from build123d import *

# Parameters (mm, degrees)
ESQUISSE1_W             = 150
ESQUISSE1_H             = 150
BOSS_EXTRU_1_DEPTH      = 250
CONG_1_R                = 20
ESQUISSE2_W             = 60
ESQUISSE2_H             = 80
ENL_V_MAT_EXTRU_1_DEPTH = 40
ESQUISSE4_W             = 60
ESQUISSE4_H             = 60
ENL_V_MAT_EXTRU_2_DEPTH = 40


with BuildPart() as part:
    # Esquisse1 → Boss.-Extru.1 (new body)
    with BuildSketch(Plane.XY):
        with Locations((75, 75)):
            Rectangle(ESQUISSE1_W, ESQUISSE1_H)
    extrude(amount=BOSS_EXTRU_1_DEPTH)

    # Congé1
    cong_1_edges = [part.edges().sort_by_distance(p)[0] for p in [
        (150, 75, 250),
        (75, 150, 250),
        (0, 75, 250),
        (75, 150, 0),
        (150, 75, 0),
        (75, 0, 0),
        (0, 75, 0),
        (0, 150, 125),
        (150, 150, 125),
        (150, 0, 125),
        (0, 0, 125),
        (75, 0, 250),
    ]]
    fillet(cong_1_edges, radius=CONG_1_R)

    # Esquisse2 → Enlèv. mat.-Extru.1 (cut)
    with BuildSketch(Plane(origin=(150, 0, 0), x_dir=(0, 0, -1), z_dir=(1, 0, 0))):
        with Locations((-105.364762055, 20.069300744)):
            Rectangle(ESQUISSE2_W, ESQUISSE2_H)
    extrude(amount=-ENL_V_MAT_EXTRU_1_DEPTH, mode=Mode.SUBTRACT)

    # Esquisse4 → Enlèv. mat.-Extru.2 (cut)
    with BuildSketch(Plane.ZY):
        with Locations((105.517882432, 30)):
            Rectangle(ESQUISSE4_W, ESQUISSE4_H)
    extrude(amount=-ENL_V_MAT_EXTRU_2_DEPTH, mode=Mode.SUBTRACT)


solid = part.part
Geometry: final body of the model. Coordinates: model frame, mm. A direction names the side the tool comes from. Give positions to 0.01 mm unless a question says otherwise; leave off trailing zeros. Loops run counter-clockwise (first coordinate to the right, second up) from the corner with the lowest first, then second, coordinate; pieces in that order, holes last. Notation, with made-up numbers: (88.25, 86) - (117.25, 86) arc R34 ccw to (117.25, 122) - close; hole circle Ø6 at (50.5, 66). An arc over 180 degrees is marked (long way). One line per question, with ' | ' between items. Start each with the question number.
(1) Ray query, line 1 (Z direction, x = 38, y = 41); line 2 (X direction, y = 14, z = 77); line 3 (Z direction, x = 15, y = 16). Return the intervals inside material, ascending. Write a range as from..to.
(2) Pull-direction query (Z, two-part tool) for faces 3 (the flat face through (74, 0, 124)), 4 (the flat face through (130, 30, 75.365)), 5 (the cylindrical face through (75.77, 5.703, 6.014)); classes: released by +Z, released by -Z, zero draft, split by the parting line, or undercut.
(3) Contact query for flat-ended pins moving along their axis: pin 1 (12 mm diameter, centred on x = 16.5, z = 93, fed in from -Y); pin 2 (1 mm diameter, centred on x = 77.5, y = 18.5, fed in from -Z) (3 decimals). Output: stop coordinate, or through.
(4) Section query D-D on z = 169.5. Return loops of the section in (x, y).
(5) Reachability of faces 1 (the flat face through (110, 30, 106)), 2 (the cylindrical face through (143.986, 5.703, 183.345)) from +Z, -Z, +X, -X, +Y, -Y: full face, straight path, thin tool, end or side. Return the list, or none.
(6) Section query B-B on x = 23. Return loops of the section in (y, z).
(7) Section query C-C on z = 113.5. Return loops of the section in (x, y), then the cut area to 3 significant figures.
(8) Section query A-A on y = 28. Return loops of the section in (x, z).
The answers:
1) line 1: 0..75.52, 135.52..250 | line 2: 40..110 | line 3: 1.05..75.52, 135.52..248.95
2) face 3: zero draft | face 4: undercut | face 5: released by -Z
3) pin 1: y = 60 | pin 2: z = 0.025
4) outline: (0, 20) arc R20 ccw to (20, 0) - (130, 0) arc R20 ccw to (150, 20) - (150, 130) arc R20 ccw to (130, 150) - (20, 150) arc R20 ccw to (0, 130) - close
5) face 1: +X, -Y | face 2: +Z, -Z, +X, -Y
6) outline: (0, 20) arc R20 ccw to (20, 0) - (130, 0) arc R20 ccw to (150, 20) - (150, 230) arc R20 ccw to (130, 250) - (20, 250) arc R20 ccw to (0, 230) - (0, 135.52) - (60, 135.52) - (60, 75.52) - (0, 75.52) - close
7) outline: (0, 60) - (40, 60) - (40, 0) - (110, 0) - (110, 60.07) - (150, 60.07) - (150, 130) arc R20 ccw to (130, 150) - (20, 150) arc R20 ccw to (0, 130) - close | area: 17,500 mm2
8) outline: (0, 20) arc R20 ccw to (20, 0) - (130, 0) arc R20 ccw to (150, 20) - (150, 75.36) - (110, 75.36) - (110, 135.36) - (150, 135.36) - (150, 230) arc R20 ccw to (130, 250) - (20, 250) arc R20 ccw to (0, 230) - (0, 135.52) - (40, 135.52) - (40, 75.52) - (0, 75.52) - close
